```python
from build123d import *

# Parameters (mm, degrees)
SKETCH1_R      = 2
EXTRUDE1_DEPTH = 3
EXTRUDE3_DEPTH = 1.82
SKETCH2_R      = 1.475
EXTRUDE2_DEPTH = 12


with BuildPart() as part:
    # Sketch1 → Extrude1 (new body)
    with BuildSketch(Plane.XY):
        Circle(SKETCH1_R)
    extrude(amount=EXTRUDE1_DEPTH)

    # Sketch3 → Extrude3 (cut)
    with BuildSketch(Plane(origin=(0, 0, 0), x_dir=(-1, 0, 0), z_dir=(0, 0, -1))):
        Polygon((-1.443375673, 0), (-0.721687836, -1.25), (0.721687836, -1.25), (1.443375673, 0), (0.721687836, 1.25), (-0.721687836, 1.25), align=None)
    extrude(amount=-EXTRUDE3_DEPTH, mode=Mode.SUBTRACT)

    # Sketch2 → Extrude2 (add)
    with BuildSketch(Plane.XY.offset(3)):
        Circle(SKETCH2_R)
    extrude(amount=EXTRUDE2_DEPTH)


solid = part.part
```
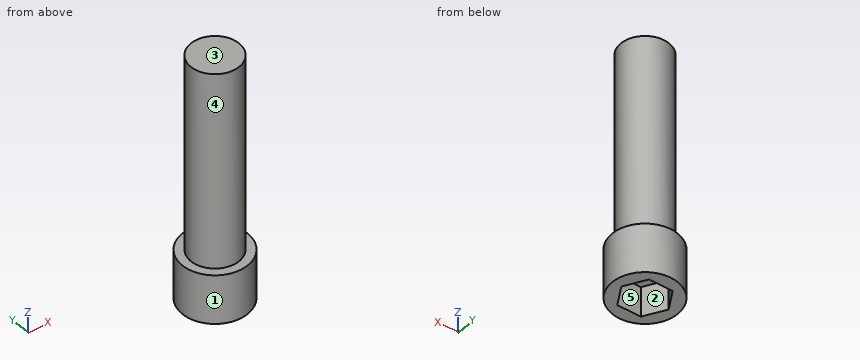
For this review, take the finished solid that the model builds, in its own axes (mm). Face numbers are marked on the shaded views. A direction names the side the tool comes from. Round coordinates to 2 decimals unless told otherwise and drop trailing zeros. Write each loop counter-clockwise with the first axis right and the second up, starting at its lowest first coordinate (ties: lowest second). Pieces come first, ordered by that corner, then holes. Notation, with made-up numbers: (-15.75, -1.5) - (13.25, -1.5) arc R15 ccw to (13.25, 11.5) - close; hole circle Ø7 at (1, 13). An arc over 180 degrees is marked (long way). Use CSV: the item, a comma, the result in double quotes.
1) For the marked faces 4 and 5, list the 3-axis set-ups (+Z, -Z, +X, -X, +Y, -Y) from which the entire face can be reached by the end or side of a thin tool; tool diameter is ignored.
Conclusion:
face 4,"+Z"
face 5,"-Z"
2) Clearance check with flat-ended pins moving along their axes: pin 1 Ø1.5 at (x, z) = (1.5, 10) entering from +Y; pin 2 Ø1.2 at (x, y) = (-0.5, 0) entering from -Z. State where each tip first meets the part, or that it passes through.
Conclusion:
pin 1,"stops at y = 1.27"
pin 2,"stops at z = 1.82"
3) Wall thickness on line 1 along Z through (x, y) = (-0.8, -1.6); line 2 along X through (y, z) = (0.65, 1.5); line 3 along Z through (x, y) = (0.6, 1.1): over which ranges is each line inside the solid? List them lowest first. Write a range as from..to.
Conclusion:
line 1,"z = 0..3"
line 2,"x = -1.89..-1.07, 1.07..1.89"
line 3,"z = 1.82..15"
4) The part is to be moulded in two halves that separate along X. For the marked faces 1, 2 and 3, say which applies: pulls with the +X half, pulls with the -X half, needs draft (parallel to the pull), parting line crosses it, or undercut.
Conclusion:
face 1,"parting line crosses it"
face 2,"undercut"
face 3,"needs draft"
5) Add section D-D on z = 9.5. Write out the cut boundary in (x, y) (3 decimals), and give its area (3 significant figures).
Conclusion:
outline,"circle Ø2.95 at (0, 0)"
area,"6.83 mm^2"
6) Add section B-B on x = 0. Write out the cut boundary in (y, z) (3 decimals), and give its area (4 significant figures).
Conclusion:
outline,"(-2, 0) - (-1.25, 0) - (-1.25, 1.82) - (1.25, 1.82) - (1.25, 0) - (2, 0) - (2, 3) - (1.475, 3) - (1.475, 15) - (-1.475, 15) - (-1.475, 3) - (-2, 3) - close"
area,"42.85 mm^2"
7) Add section A-A on z = 1.5. Write out the cut boundary in (x, y).
Conclusion:
outline,"circle Ø4 at (0, 0); hole (-1.44, 0) - (-0.72, -1.25) - (0.72, -1.25) - (1.44, 0) - (0.72, 1.25) - (-0.72, 1.25) - close"
8) Add section C-C on y = -1. Write out the cut boundary in (x, z), and give its area (3 significant figures).
Conclusion:
outline,"(-1.73, 0) - (-0.87, 0) - (-0.87, 1.82) - (0.87, 1.82) - (0.87, 0) - (1.73, 0) - (1.73, 3) - (1.08, 3) - (1.08, 15) - (-1.08, 15) - (-1.08, 3) - (-1.73, 3) - close"
area,"33.3 mm^2"
